Could you check a few things on this model? Use its own coordinates, in mm. A direction names the side the tool comes from. Round coordinates to 2 decimals unless told otherwise and drop trailing zeros. Loops run counter-clockwise (first coordinate to the right, second up) from the corner with the lowest first, then second, coordinate; pieces in that order, holes last. Notation, with made-up numbers: (-39, 13) -> (-29, 13) arc R9 cw to (-29, 28) -> close; hole circle Ø7 at (-8.75, 57). An arc over 180 degrees is marked (long way). Write each question's results on one line, items separated by ' | '. Start each with the question number.
1) Imagine slicing it at D-D, the plane y = 6.75. List the corners of the cut face in (x, z) for me, plus the area to 3 significant figures.
2) Imagine slicing it at C-C, the plane x = -14.75. List the corners of the cut face in (y, z) for me, plus the area to 3 significant figures.
3) Which directions (+Z, -Z, +X, -X, +Y, -Y) give clear straight access to the entire face, cutting with the end or side of a thin tool? Please do faces 1 (the flat face through (-6, 5.08, 13)), 2 (the cylindrical face through (-18.856, 4.107, 6.568)), 3 (the flat face through (-11.176, 3, 6)).
4) Imagine slicing it at A-A, the plane z = 16. List the corners of the cut face in (x, y) for me, plus the area to 3 significant figures.
5) If I drill on probe 1 along Z at (x, y) = (-7.75, 1.5); probe 2 along Y at (x, z) = (-0.75, 8.5); probe 3 along Z at (x, y) = (-13.5, 5.5), over which ranges is the centre line in solid material (lowest first)?
6) Imagine slicing it at B-B, the plane y = 2. List the corners of the cut face in (x, z) for me, plus the area to 3 significant figures.
7) For P1, Ø1.5, axis at y = 3, z = 9, coming from the -X side; P2, Ø1.5, axis at y = 2.5, z = 10.5, coming from the -X side; P3, Ø6, axis at x = -2.5, z = 19, coming from the +Y side, each with a flat end and sliding along its axis, tell me the tip position at first contact or that it passes through.
8) We'd pull the mould along X, two halves only. Please class faces 4 (the cylindrical face through (-8.38, 2.58, 17.59)), 5 (the flat face through (0, 3, 13)), 6 (the cylindrical face through (-20.22, 8.55, 19.09)), 7 (the flat face through (-6, 0, 15)): pulls with the +X half, pulls with the -X half, needs draft (parallel to the pull), parting line crosses it, or undercut.
from build123d import *

# Parameters (mm, degrees)
BOSS_EXTRUDE1_DEPTH = 25.4
SKETCH5_R           = 2.286
CUT_EXTRUDE3_DEPTH  = 12.954
SKETCH8_R           = 5.334
CUT_EXTRUDE5_DEPTH  = 12.954
SKETCH9_R           = 2.54
BOSS_EXTRUDE2_DEPTH = 12.954
CUT_EXTRUDE7_DEPTH  = 12.954


with BuildPart() as part:
    # Sketch2 → Boss-Extrude1 (new body)
    with BuildSketch(Plane.XY):
        with BuildLine():
            Line((0, 0), (-16.51, 0))
            ThreePointArc((-16.51, 0), (-20.102102448, 8.672102448), (-11.43, 5.08))
            Line((-11.43, 5.08), (0, 5.08))
            Line((0, 5.08), (0, 0))
        make_face()
    extrude(amount=BOSS_EXTRUDE1_DEPTH)

    # Sketch5 → Cut-Extrude3 (cut)
    with BuildSketch(Plane(origin=(0, 5.08, 0), x_dir=(1, 0, 0), z_dir=(0, 1, 0))):
        with Locations((-6.096, -17.695333333)):
            Circle(SKETCH5_R)
        with Locations((-6.096, -7.704666667)):
            Circle(SKETCH5_R)
    extrude(amount=-CUT_EXTRUDE3_DEPTH, mode=Mode.SUBTRACT)

    # Sketch8 → Cut-Extrude5 (cut)
    with BuildSketch(Plane(origin=(0, 0, 0), x_dir=(-1, 0, 0), z_dir=(0, 0, -1))):
        with Locations((16.51, 5.08)):
            Circle(SKETCH8_R)
    extrude(amount=-CUT_EXTRUDE5_DEPTH, mode=Mode.SUBTRACT)

    # Sketch9 → Boss-Extrude2 (add)
    with BuildSketch(Plane(origin=(0, 0, 12.954), x_dir=(-1, 0, 0), z_dir=(0, 0, -1))):
        with Locations((16.51, 5.08)):
            Circle(SKETCH9_R)
    extrude(amount=BOSS_EXTRUDE2_DEPTH)

    # Sketch10 → Cut-Extrude7 (cut)
    with BuildSketch(Plane(origin=(0, 0, 0), x_dir=(-1, 0, 0), z_dir=(0, 0, -1))):
        with BuildLine():
            Line((11.176, 5.08), (11.176, 0))
            Line((11.176, 0), (14.883606444, 0))
            ThreePointArc((14.883606444, 0), (12.201477096, 1.935451322), (11.176, 5.08))
        make_face()
    extrude(amount=-CUT_EXTRUDE7_DEPTH, mode=Mode.SUBTRACT)


solid = part.part
Checked values:
1) outline: (-21.31, 12.95) -> (-18.42, 12.95) -> (-18.42, 0) -> (-14.6, 0) -> (-14.6, 12.95) -> (-11.71, 12.95) -> (-11.71, 25.4) -> (-21.31, 25.4) -> close | area: 169 mm^2
2) outline: (0, 12.95) -> (3.25, 12.95) -> (3.25, 0) -> (6.91, 0) -> (6.91, 12.95) -> (9.85, 12.95) -> (9.85, 25.4) -> (0, 25.4) -> close | area: 170 mm^2
3) face 1: +Z, -Z, +X, +Y | face 2: -Z | face 3: -Z, +Y, -Y
4) outline: (-16.51, 0) -> (-7.63, 0) -> (-7.63, 5.08) -> (-11.43, 5.08) arc R5.08 ccw (long way) to start; (-4.56, 0) -> (0, 0) -> (0, 5.08) -> (-4.56, 5.08) -> close | area: 129 mm^2
5) probe 1: 0 to 6.13, 9.28 to 16.12, 19.27 to 25.4 | probe 2: 0 to 5.08 | probe 3: 12.95 to 25.4
6) outline: (-20.55, 12.95) -> (-11.18, 12.95) -> (-11.18, 0) -> (0, 0) -> (0, 25.4) -> (-20.55, 25.4) -> close; hole circle Ø4.57 at (-6.1, 7.7); hole circle Ø4.57 at (-6.1, 17.7) | area: 368 mm^2
7) P1: x = -18.67 | P2: x = -18.27 | P3: y = 5.08
8) face 4: undercut | face 5: pulls with the +X half | face 6: parting line crosses it | face 7: needs draft
